Verification items for the finished model (mm, model axes). A direction names the side the tool comes from. Round coordinates to 2 decimals unless told otherwise and drop trailing zeros. Write each loop counter-clockwise with the first axis right and the second up, starting at its lowest first coordinate (ties: lowest second). Pieces come first, ordered by that corner, then holes. Notation, with made-up numbers: M 16.5,85.25 L 49.5,85.25 A19 ccw 49.5,99.25 Z; hole C 62,23 d2. An arc over 180 degrees is marked long. Use a Markdown table: item, result. Add a question column.
from build123d import *

# Parameters (mm, degrees)
BOSS_EXTRUDE2_DEPTH = 32
CUT_EXTRUDE2_DEPTH  = 21
CUT_EXTRUDE3_DEPTH  = 21
CUT_EXTRUDE4_DEPTH  = 5
CUT_EXTRUDE5_DEPTH  = 5
CUT_EXTRUDE6_REACH  = 17
CUT_EXTRUDE7_REACH  = 102


with BuildPart() as part:
    # Sketch1 → Boss-Extrude2 (new body, symmetric)
    with BuildSketch(Plane.XY):
        Polygon((-13.146933892, 26.49867374), (56.853066108, -13.50132626), (-13.146933892, -13.50132626), align=None)
        Polygon((-13.146933892, 26.49867374), (-13.146933892, -13.50132626), (56.853066108, -13.50132626), (71.853066108, -13.50132626), (71.853066108, -35.50132626), (-28.146933892, -35.50132626), (-28.146933892, 39.49867374), (-13.146933892, 39.49867374), align=None)
    extrude(amount=BOSS_EXTRUDE2_DEPTH, both=True)

    # Sketch3 → Cut-Extrude2 (cut)
    with BuildSketch(Plane.XY.offset(32)):
        Polygon((-13.146933892, 26.49867374), (-13.146933892, -13.50132626), (56.853066108, -13.50132626), align=None)
    extrude(amount=-CUT_EXTRUDE2_DEPTH, mode=Mode.SUBTRACT)

    # Sketch4 → Cut-Extrude3 (cut)
    with BuildSketch(Plane(origin=(0, 0, -32), x_dir=(-1, 0, 0), z_dir=(0, 0, -1))):
        Polygon((13.146933892, 26.49867374), (13.146933892, -13.50132626), (-56.853066108, -13.50132626), align=None)
    extrude(amount=-CUT_EXTRUDE3_DEPTH, mode=Mode.SUBTRACT)

    # Sketch8 → Cut-Extrude4 (cut)
    with BuildSketch(Plane.XY.offset(11)):
        Polygon((-13.146933892, 26.49867374), (56.853066108, -13.50132626), (-13.146933892, -13.50132626), align=None)
    extrude(amount=-CUT_EXTRUDE4_DEPTH, mode=Mode.SUBTRACT)

    # Sketch9 → Cut-Extrude5 (cut)
    with BuildSketch(Plane(origin=(0, 0, -11), x_dir=(-1, 0, 0), z_dir=(0, 0, -1))):
        Polygon((13.146933892, 26.49867374), (-56.853066108, -13.50132626), (13.146933892, -13.50132626), align=None)
    extrude(amount=-CUT_EXTRUDE5_DEPTH, mode=Mode.SUBTRACT)

    # Sketch10 → Cut-Extrude6 (cut, up to next)
    with BuildSketch(Plane(origin=(-13.146933892, 0, 0), x_dir=(0, 0, -1), z_dir=(1, 0, 0)), mode=Mode.PRIVATE) as cut_extrude6_sk1:
        Polygon((-16, 39.49867374), (-32, 39.49867374), (-32, 24.946500862), align=None)
    cut_extrude6_tool1 = extrude(cut_extrude6_sk1.sketch, amount=-CUT_EXTRUDE6_REACH, mode=Mode.PRIVATE) & part.part
    add(cut_extrude6_tool1.solids().sort_by_distance((-13.146934, 34.647949, 26.666667))[0], mode=Mode.SUBTRACT)
    # Sketch10 → Cut-Extrude6 (cut, up to next)
    with BuildSketch(Plane(origin=(-13.146933892, 0, 0), x_dir=(0, 0, -1), z_dir=(1, 0, 0)), mode=Mode.PRIVATE) as cut_extrude6_sk2:
        Polygon((32, 39.49867374), (16, 39.49867374), (32, 24.946500862), align=None)
    cut_extrude6_tool2 = extrude(cut_extrude6_sk2.sketch, amount=-CUT_EXTRUDE6_REACH, mode=Mode.PRIVATE) & part.part
    add(cut_extrude6_tool2.solids().sort_by_distance((-13.146934, 34.647949, -26.666667))[0], mode=Mode.SUBTRACT)

    # Sketch11 → Cut-Extrude7 (cut, up to next)
    with BuildSketch(Plane(origin=(71.853066108, 0, 0), x_dir=(0, 0, -1), z_dir=(1, 0, 0)), mode=Mode.PRIVATE) as cut_extrude7_sk1:
        Polygon((-8.07179677, -35.50132626), (8.07179677, -35.50132626), (15, -23.50132626), (-15, -23.50132626), align=None)
    cut_extrude7_tool1 = extrude(cut_extrude7_sk1.sketch, amount=-CUT_EXTRUDE7_REACH, mode=Mode.PRIVATE) & part.part
    add(cut_extrude7_tool1.solids().sort_by_distance((71.853066, -28.900749, 0))[0], mode=Mode.SUBTRACT)


solid = part.part
1. Cross-section at B-B on z = -12. Enter the section's corners in (x, y), plus the area to 3 significant figures.
2. Access from +Z, -Z, +X, -X, +Y, -Y to the whole of each face (thin tool, end or side, straight path). Record for faces 5 (the flat face through (22.553, -29.417, 11.584)), 6 (the flat face through (7, -2, -6)), 7 (the flat face through (7, -2, 6)), 8 (the flat face through (-13.147, 13, 8)), 9 (the flat face through (11, -18, -32)).
3. Cross-section at C-C on y = -8.5. Enter the section's corners in (x, z).
4. Cross-section at D-D on z = 10. Enter the section's corners in (x, y).
5. Cross-section at A-A on x = -21. Enter the section's corners in (y, z).
6. Release check for a two-part mould opening along Y. For faces 1 (the flat face through (21.36, 6.78, 0.08)), 2 (the flat face through (23, -35.501, 20)), 3 (the flat face through (11, -18, 32)), 4 (the flat face through (23, -23.501, 0)) record: +Y half, -Y half, draft (parallel to the pull), parting line (faces both ways), or undercut.
7. Scan lines: line 1 along X through (y, z) = (4, -16.5); line 2 along Y through (x, z) = (17, -29); line 3 along Z through (x, y) = (-13, 21.5). Record each from-to range of solid material in increasing order. Write a range as from..to.
8. Depth check by flat-ended pin: pin 1 Ø12 at (x, y) = (38, -1) entering from -Z; pin 2 Ø12 at (y, z) = (6.5, 14.5) entering from +X; pin 3 Ø1 at (x, y) = (6.5, -11.5) entering from +Z. Enter the tip coordinate at first touch or a pass-through.
Answer:
| question | item | result |
|---|---|---|
| 1 | outline | M -28.15,-35.5 L 71.85,-35.5 L 71.85,-28.7 L -28.15,-28.7 Z; M -28.15,-23.5 L 71.85,-23.5 L 71.85,-13.5 L -13.15,-13.5 L -13.15,39.5 L -28.15,39.5 Z |
| 1 | area | 2,480 mm^2 |
| 2 | face 5 | +X, -X |
| 2 | face 6 | -Z, +X, +Y |
| 2 | face 7 | +Z, +X, +Y |
| 2 | face 8 | +X, +Y |
| 2 | face 9 | -Z, +X, -X, +Y, -Y |
| 3 | outline | M -28.15,-32 L -13.15,-32 L -13.15,-6 L 48.1,-6 L 48.1,6 L -13.15,6 L -13.15,32 L -28.15,32 Z |
| 4 | outline | M -28.15,-35.5 L 71.85,-35.5 L 71.85,-32.16 L -28.15,-32.16 Z; M -28.15,-23.5 L 71.85,-23.5 L 71.85,-13.5 L -13.15,-13.5 L -13.15,39.5 L -28.15,39.5 Z |
| 5 | outline | M -35.5,-32 L 24.95,-32 L 39.5,-16 L 39.5,16 L 24.95,32 L -35.5,32 L -35.5,8.07 L -23.5,15 L -23.5,-15 L -35.5,-8.07 Z |
| 6 | face 1 | +Y half |
| 6 | face 2 | -Y half |
| 6 | face 3 | draft |
| 6 | face 4 | undercut |
| 7 | line 1 | x = -28.15..-13.15 |
| 7 | line 2 | y = -35.5..-13.5 |
| 7 | line 3 | z = -6..6 |
| 8 | pin 1 | stops at z = -6 |
| 8 | pin 2 | stops at x = -13.15 |
| 8 | pin 3 | stops at z = 6 |
